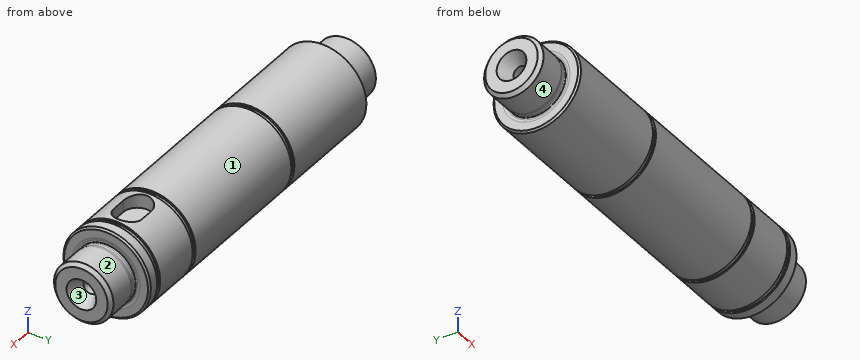
Autodesk Inventor part; units mm, degrees
ref_plane "Work Plane1" through (0, 0, 12.5) normal (0, 0, 1) x (1, 0, 0)
ref_plane "YZ Plane" through (0, 0, 0) normal (1, 0, 0) x (0, 1, 0)
ref_plane "XZ Plane" through (0, 0, 0) normal (0, 1, 0) x (-1, 0, 0)
sketch "Sketch1" plane through (0, 0, 0) normal (0, 1, 0) x (-1, 0, 0)
  line L0 (0, 0) -> (93.8, 0)
  line L1 (0, 9.695) -> (0.1, 8.9835)
  line L2 (0, 12.5) -> (0, 9.695)
  line L3 (3.2, 12.5) -> (0, 12.5)
  line L4 (3.2, 11.95) -> (3.2, 12.5)
  line L5 (4.5, 11.95) -> (3.2, 11.95)
  line L6 (4.5, 12.5) -> (4.5, 11.95)
  line L7 (18.5, 12.5) -> (4.5, 12.5)
  line L8 (18.5, 11.95) -> (18.5, 12.5)
  line L9 (19.8, 11.95) -> (18.5, 11.95)
  line L10 (19.8, 12.5) -> (19.8, 11.95)
  line L11 (61, 12.5) -> (19.8, 12.5)
  line L12 (61, 11.95) -> (61, 12.5)
  line L13 (62.3, 11.95) -> (61, 11.95)
  line L14 (62.3, 12.5) -> (62.3, 11.95)
  line L15 (93.8, 12.5) -> (62.3, 12.5)
  line L16 (93.8, 9.695) -> (93.8, 12.5)
  line L17 (93.7, 8.9835) -> (93.8, 9.695)
  line L18 (93.8, 0) -> (93.8, 8.5597)
  line L19 (0, 0) -> (93.8, 0)
  line L20 (0, 8.5597) -> (0, 0)
  arc A0 (0, 8.5597) -> (0.1, 8.9835) centre (-0.4942, 8.9) ccw
  arc A1 (93.7, 8.9835) -> (93.8, 8.5597) centre (94.2942, 8.9) ccw
  dimension "d0" = 0
  dimension "d1" = 12.5
  dimension "d2" = 8.5597
  dimension "d3" = 2.805
  dimension "d4" = 0.7185
  dimension "d5" = 0.6
  dimension "d6" = 3.2
  dimension "d7" = 0.55
  dimension "d8" = 1.3
  dimension "d9" = 0.55
  dimension "d10" = 14
  dimension "d11" = 0.55
  dimension "d12" = 1.3
  dimension "d13" = 0.55
  dimension "d14" = 41.2
  dimension "d15" = 0.55
  dimension "d16" = 1.3
  dimension "d17" = 0.55
  dimension "d18" = 31.5
  dimension "d19" = 2.805
  dimension "d20" = 0.7115
  dimension "d21" = 0.6
  dimension "d22" = 8.5597
  dimension "d23" = 93.8
  dimension "d24" = 90
  dimension "d25" = 90
  dimension "d26" = 90
  dimension "d27" = 90
  dimension "d28" = 90
  dimension "d29" = 90
  dimension "d30" = 90
  dimension "d31" = 90
  dimension "d32" = 90
  dimension "d33" = 90
revolve "Revolution1" add sketch "Sketch1" angle 360 about axis through (0, 0, 0) along (-1, 0, 0)
sketch "Sketch2" plane through (0, 0, 0) normal (0, 0, 1) x (1, 0, 0)
  line L0 (0, 0) -> (-0.1, 8.4994)
  line L1 (0, 0) -> (-0.01, 8.5)
  line L2 (-0.01, 8.5) -> (0.04, 8.5)
  line L3 (0.04, 8.5) -> (0.04, 8.3) construction
  line L4 (0.04, 8.3) -> (0.49, 8.3) construction
  arc A0 (0.04, 8.5) -> (0.49, 8.3) centre (0.4872, 8.9) ccw
  line L5 (0.49, 8.3) -> (1.25, 8.3)
  line L6 (1.25, 8.3) -> (2, 8.3) construction
  line L7 (2, 8.3) -> (2, 8.5) construction
  line L8 (2, 8.5) -> (10.6, 8.5)
  line L9 (10.6, 8.5) -> (10.6, 0)
  line L10 (10.6, 0) -> (0, 0)
  line L11 (-19.8, 12.5) -> (-61, 12.5)
  line L12 (-40.4, 12.5) -> (-40.4, -12.5)
  line L13 (-19.8, -12.5) -> (-61, -12.5)
  line L14 (-46.9, 25.3625) -> (-46.9, -42.5251)
  line L15 (-93.8, 12.5) -> (-93.8, -12.5)
  line L16 (2, 8.5) -> (1.25, 8.3)
  line L17 (-93.8, 0) -> (-93.79, 8.5)
  line L18 (-93.79, 8.5) -> (-93.84, 8.5)
  line L19 (-93.84, 8.5) -> (-93.84, 8.3) construction
  line L20 (-93.84, 8.3) -> (-94.29, 8.3) construction
  arc A1 (-94.29, 8.3) -> (-93.84, 8.5) centre (-94.2872, 8.9) ccw
  line L21 (-94.29, 8.3) -> (-95.05, 8.3)
  line L22 (-95.05, 8.3) -> (-95.8, 8.3) construction
  line L23 (-95.8, 8.3) -> (-95.8, 8.5) construction
  line L24 (-95.8, 8.5) -> (-104.4, 8.5)
  line L25 (-104.4, 8.5) -> (-104.4, 0)
  line L26 (-104.4, 0) -> (-93.8, 0)
  line L27 (-95.8, 8.5) -> (-95.05, 8.3)
  dimension "d35" = 8.5
  dimension "d36" = 8.5
  dimension "d37" = 0.05
  dimension "d38" = 0.2
  dimension "d39" = 0.45
  dimension "d40" = 0.6
  dimension "d41" = 0.76
  dimension "d42" = 0.75
  dimension "d43" = 0.2
  dimension "d44" = 8.6
  dimension "d45" = 90
  dimension "d60" = 10.6
  dimension "d61" = 0
revolve "Revolution2" add sketch "Sketch2" angle 360 about axis through (10.6, 0, 0) along (-1, 0, 0) contours L1 L2 A0 L5 L16 L8 L9 L10 | L18 L17 L15 | L15 L26 L25 L24 L27 L21 A1 L18
chamfer "Chamfer1" distance 1 angle 45 1 edges at (10.6, -8.5, 0) measured on face at (4.8667, 8.4724, 0.684)
chamfer "Chamfer2" distance 1 angle 45 1 edges at (-104.4, -8.5, 0) measured on face at (-98.6667, 8.4724, 0.684)
chamfer "Chamfer3" distance 0.5 angle 45 1 edges at (0, 0, -12.5) measured on face at (-2.1333, -2.0051, 12.3381)
chamfer "Chamfer4" distance 0.5 angle 45 1 edges at (-93.8, 0, -12.5) measured on face at (-83.3, -1.0058, 12.4595)
sketch "Sketch3" plane through (0, 0, 0) normal (0, 0, 1) x (1, 0, 0)
  point P0 (0, 0)
ref_plane "Work Plane1" through (0, 0, 12.5) normal (0, 0, 1) x (1, 0, 0)
sketch "Sketch4" plane through (0, 0, 12.5) normal (0, 0, 1) x (1, 0, 0)
  line L0 (-13.5, 0) -> (-9.5, 0) construction
  line L1 (-13.5, 4) -> (-9.5, 4)
  line L2 (-9.5, -4) -> (-13.5, -4)
  arc A0 (-13.5, 4) -> (-13.5, -4) centre (-13.5, 0) ccw
  arc A1 (-9.5, -4) -> (-9.5, 4) centre (-9.5, 0) ccw
  line L3 (10.6, 7.5) -> (10.6, -7.5)
  point P0 (0, 0)
  point P1 (-11.5, 0)
  point P2 (-5.5, 0)
  point P3 (-17.5, 0)
  dimension "d63" = 12
  dimension "d64" = 8
  dimension "d65" = 16.1
  dimension "d66" = 0
extrude "Extrusion1" cut sketch "Sketch4" against normal blind 4
sketch "Sketch5" plane through (10.6, 0, 0) normal (1, 0, 0) x (0, 0, -1)
  point P0 (0, 0)
hole "Hole1" at (10.6, 0, 0) direction (-1, 0, 0) diameter 4 depth 6.47 tip angle 118 countersink diameter 8.5 countersink angle 60
sketch "Sketch6" plane through (-104.4, 0, 0) normal (-1, 0, 0) x (0, 0, 1)
  point P0 (0, 0)
hole "Hole2" at (-104.4, 0, 0) direction (1, 0, 0) diameter 4 depth 6.47 tip angle 118 countersink diameter 8.5 countersink angle 60
properties part number "26-10-204"
Can you work these out from the model? Positions are in its coordinate system, mm. Face numbers are marked on the shaded views. A direction names the side the tool comes from. Round coordinates to 2 decimals unless told otherwise and drop trailing zeros. Order: outer loops, then holes, each group sorted by start corner. A loop starts at its lowest first (then second) coordinate and runs counter-clockwise, first axis right, second up. Notation, with made-up numbers: M 0,49.25 L 51,49.25 A22 ccw 51,76.25 Z; hole C 52.5,40.5 d10. An arc over 180 degrees is marked long. Use a Markdown table: item, result.
1) If we mould it in two halves opening along Y, with no side actions, what happens to the marked faces 3 and 4? For each: +Y half, -Y half, draft (parallel to the pull), parting line (faces both ways), or undercut.
Geometry says:
| item | result |
|---|---|
| face 3 | undercut |
| face 4 | parting line |
2) Imagine slicing it at A-A (x = -65). List the corners of the cut face in (y, z) for me.
Geometry says:
| item | result |
|---|---|
| outline | C 0,0 d25 |
3) If I drill on line 1 along Y through (x, z) = (5.2, 0); line 2 along X through (y, z) = (-10.75, -2), over which ranges is the centre line in solid material (lowest first)?
Geometry says:
| item | result |
|---|---|
| line 1 | y = -8.5 to -2, 2 to 8.5 |
| line 2 | x = -93.8 to 0 |
4) On a 3-axis mill with a long thin cutter (end or side, diameter ignored), from which of +Z, -Z, +X, -X, +Y, -Y can I reach the whole of each face in a straight line? I mean the marked faces 1 and 2. Say none if no direction works.
Geometry says:
| item | result |
|---|---|
| face 1 | +X, -X |
| face 2 | +X |
5) I'm going to push flat-ended pins straight in: P1, Ø4.5, axis at y = 0, z = 0, coming from the +X side; P2, Ø8, axis at y = -8, z = 8.5, coming from the +X side; P3, Ø6.5, axis at x = -12, y = -1.5, coming from the +Z side. Where does each tip first touch, or does it pass through?
Geometry says:
| item | result |
|---|---|
| P1 | stops at x = 7.14 |
| P2 | stops at x = 10.43 |
| P3 | stops at z = 11.86 |
